Model file for the job. Use its own axes, mm. Face numbers are marked on the shaded views. A direction names the side the tool comes from. Round coordinates to 2 decimals unless told otherwise and drop trailing zeros. Loops run counter-clockwise (first coordinate to the right, second up) from the corner with the lowest first, then second, coordinate; pieces in that order, holes last. Notation, with made-up numbers: (-4.75, 65.5) - (46.25, 65.5) arc R14 cw to (46.25, 81.5) - close; hole circle Ø5 at (85.5, -22.75). An arc over 180 degrees is marked (long way). Answer as a JSON object with one key per item and string values.
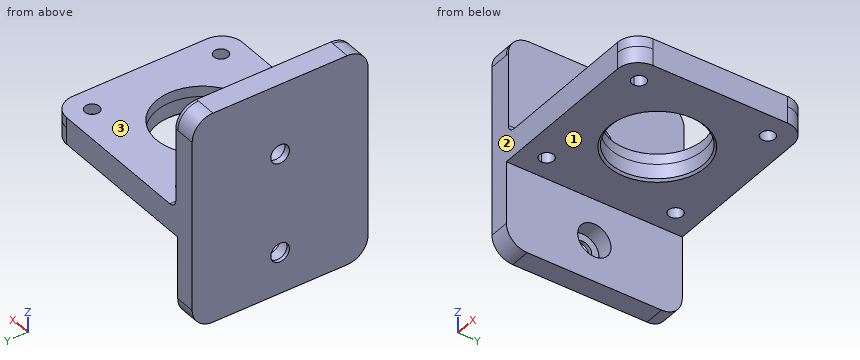
from build123d import *

# Parameters (mm, degrees)
SKETCH1_W                      = 42.3
SKETCH1_H                      = 42.3
BOSS_EXTRUDE1_DEPTH            = 2
M3_CLEARANCE_HOLE1_D           = 3.4
M3_CLEARANCE_HOLE1_CSINK_D     = 3.45
M3_CLEARANCE_HOLE1_CSINK_ANGLE = 90
SKETCH6_R                      = 11.125
CUT_EXTRUDE1_DEPTH             = 5
SKETCH9_W                      = 4.85
SKETCH9_H                      = 42.3
BOSS_EXTRUDE2_DEPTH            = 15
FILLET2_R                      = 5
SKETCH13_W                     = 4.85
SKETCH13_H                     = 42.3
BOSS_EXTRUDE4_DEPTH            = 7
SKETCH14_W                     = 4.85
SKETCH14_H                     = 42.3
BOSS_EXTRUDE5_DEPTH            = 14
CBORE_FOR_M4_SHCS1_D           = 4.5
CBORE_FOR_M4_SHCS1_CBORE_D     = 8
CBORE_FOR_M4_SHCS1_CBORE_DEPTH = 4
FILLET3_R                      = 5
SKETCH19_R                     = 11.125
SKETCH19_R_2                   = 1.725
SKETCH19_R_3                   = 1.7
BOSS_EXTRUDE6_DEPTH            = 2.5
BOSS_EXTRUDE6_DEPTH_BACK       = 4
BOSS_EXTRUDE7_DEPTH            = 0.65
CBORE_FOR_M4_SHCS3_D           = 4.5
CBORE_FOR_M4_SHCS3_CBORE_D     = 8
CBORE_FOR_M4_SHCS3_CBORE_DEPTH = 4
FILLET6_R                      = 2
CHAMFER1_SIZE                  = 0.5


with BuildPart() as part:
    # Sketch1 → Boss-Extrude1 (new body, symmetric)
    with BuildSketch(Plane.XY):
        Rectangle(SKETCH1_W, SKETCH1_H)
    extrude(amount=BOSS_EXTRUDE1_DEPTH, both=True)

    # M3 Clearance Hole1 (through all)
    with Locations(Plane.XY.offset(2)):
        with Locations((-15.5, 15.5), (15.5, 15.5), (15.5, -15.5), (-15.5, -15.5)):
            CounterSinkHole(M3_CLEARANCE_HOLE1_D / 2, M3_CLEARANCE_HOLE1_CSINK_D / 2, counter_sink_angle=M3_CLEARANCE_HOLE1_CSINK_ANGLE)

    # Sketch6 → Cut-Extrude1 (cut, through all)
    with BuildSketch(Plane.XY.offset(2)):
        Circle(SKETCH6_R)
    extrude(amount=-CUT_EXTRUDE1_DEPTH, mode=Mode.SUBTRACT)

    # Sketch9 → Boss-Extrude2 (add, symmetric)
    with BuildSketch(Plane.XY):
        with Locations((-23.575, 0)):
            Rectangle(SKETCH9_W, SKETCH9_H)
    extrude(amount=BOSS_EXTRUDE2_DEPTH, both=True)

    # Fillet2
    fillet2_edges = [part.edges().sort_by_distance(p)[0] for p in [
        (21.15, -21.15, 0),
        (21.15, 21.15, 0),
    ]]
    fillet(fillet2_edges, radius=FILLET2_R)

    # Sketch13 → Boss-Extrude4 (add)
    with BuildSketch(Plane(origin=(0, 0, -15), x_dir=(-1, 0, 0), z_dir=(0, 0, -1))):
        with Locations((23.575, 0)):
            Rectangle(SKETCH13_W, SKETCH13_H)
    extrude(amount=BOSS_EXTRUDE4_DEPTH)

    # Sketch14 → Boss-Extrude5 (add)
    with BuildSketch(Plane.XY.offset(15)):
        with Locations((-23.575, 0)):
            Rectangle(SKETCH14_W, SKETCH14_H)
    extrude(amount=BOSS_EXTRUDE5_DEPTH)

    # CBORE for M4 SHCS1 (through all)
    with Locations(Plane(origin=(-21.15, 0, 0), x_dir=(0, 0, -1), z_dir=(1, 0, 0))):
        with Locations((12, 0)):
            CounterBoreHole(CBORE_FOR_M4_SHCS1_D / 2, CBORE_FOR_M4_SHCS1_CBORE_D / 2, CBORE_FOR_M4_SHCS1_CBORE_DEPTH)

    # Fillet3
    fillet3_edges = [part.edges().sort_by_distance(p)[0] for p in [
        (-23.575, 21.15, -22),
        (-23.575, -21.15, -22),
        (-23.575, -21.15, 29),
        (-23.575, 21.15, 29),
    ]]
    fillet(fillet3_edges, radius=FILLET3_R)

    # Sketch19 → Boss-Extrude6 (add, two sides)
    with BuildSketch(Plane.XY.offset(2)) as boss_extrude6_sk:
        with BuildLine():
            Line((-21.15, -21.15), (16.15, -21.15))
            ThreePointArc((16.15, -21.15), (19.685533906, -19.685533906), (21.15, -16.15))
            Line((21.15, -16.15), (21.15, 16.15))
            ThreePointArc((21.15, 16.15), (19.685533906, 19.685533906), (16.15, 21.15))
            Line((16.15, 21.15), (-21.15, 21.15))
            Line((-21.15, 21.15), (-21.15, -21.15))
        make_face()
        Circle(SKETCH19_R, mode=Mode.SUBTRACT)
        with Locations((15.5, 15.5)):
            Circle(SKETCH19_R_2, mode=Mode.SUBTRACT)
        with Locations((-15.5, 15.5)):
            Circle(SKETCH19_R_2, mode=Mode.SUBTRACT)
        with Locations((-15.5, -15.5)):
            Circle(SKETCH19_R_3, mode=Mode.SUBTRACT)
        with Locations((15.5, -15.5)):
            Circle(SKETCH19_R_3, mode=Mode.SUBTRACT)
    extrude(amount=BOSS_EXTRUDE6_DEPTH)
    extrude(boss_extrude6_sk.sketch, amount=-BOSS_EXTRUDE6_DEPTH_BACK)

    # Sketch21 → Boss-Extrude7 (add)
    with BuildSketch(Plane(origin=(-21.15, 0, 0), x_dir=(0, 0, -1), z_dir=(1, 0, 0))):
        with BuildLine():
            Line((-24, -21.15), (-4.5, -21.15))
            Line((-4.5, -21.15), (-4.5, 21.15))
            Line((-4.5, 21.15), (-24, 21.15))
            ThreePointArc((-24, 21.15), (-27.535533906, 19.685533906), (-29, 16.15))
            Line((-29, 16.15), (-29, -16.15))
            ThreePointArc((-29, -16.15), (-27.535533906, -19.685533906), (-24, -21.15))
        make_face()
    extrude(amount=BOSS_EXTRUDE7_DEPTH)

    # CBORE for M4 SHCS3 (through all)
    with Locations(Plane(origin=(-20.5, 0, 0), x_dir=(0, 0, -1), z_dir=(1, 0, 0))):
        with Locations((-12, 0)):
            CounterBoreHole(CBORE_FOR_M4_SHCS3_D / 2, CBORE_FOR_M4_SHCS3_CBORE_D / 2, CBORE_FOR_M4_SHCS3_CBORE_DEPTH)

    # Fillet6
    fillet6_edges = [part.edges().sort_by_distance(p)[0] for p in [
        (-20.5, 0, 4.5),
    ]]
    fillet(fillet6_edges, radius=FILLET6_R)

    # Chamfer1
    chamfer1_edges = [part.edges().sort_by_distance(p)[0] for p in [
        (-11.125, 0, -2),
    ]]
    chamfer(chamfer1_edges, length=CHAMFER1_SIZE)


solid = part.part
1) Slice it at D-D on y = -13. List the corners of the cut face in (x, z).
Values follow:
{"outline": "(-26, -22) - (-21.15, -22) - (-21.15, -2) - (21.15, -2) - (21.15, 4.5) - (-18.5, 4.5) arc R2 cw to (-20.5, 6.5) - (-20.5, 29) - (-26, 29) - close"}
2) Slice it at C-C on z = -12. List the corners of the cut face in (x, y).
Values follow:
{"outline": "(-26, -21.15) - (-21.15, -21.15) - (-21.15, -4) - (-25.15, -4) - (-25.15, -2.25) - (-26, -2.25) - close; (-26, 2.25) - (-25.15, 2.25) - (-25.15, 4) - (-21.15, 4) - (-21.15, 21.15) - (-26, 21.15) - close"}
3) Tool access for the marked faces 1, 2 and 3: list every direction of +Z, -Z, +X, -X, +Y, -Y with a clear straight run to the whole face (end or side of a thin tool).
Values follow:
{"face 1": "-Z, +X, +Y, -Y", "face 2": "+Z, -Z, +X, -X, -Y", "face 3": "+Z, +X, +Y, -Y"}
4) Slice it at A-A on z = 12. List the corners of the cut face in (x, y).
Values follow:
{"outline": "(-26, -21.15) - (-20.5, -21.15) - (-20.5, -4) - (-24.5, -4) - (-24.5, -2.25) - (-26, -2.25) - close; (-26, 2.25) - (-24.5, 2.25) - (-24.5, 4) - (-20.5, 4) - (-20.5, 21.15) - (-26, 21.15) - close"}
5) Drop flat-ended pins along their axis: P1, Ø10, axis at y = 7.5, z = -14, coming from the +X side; P2, Ø1.5, axis at x = 9, y = 2, coming from the +Z side; P3, Ø6.5, axis at y = -0.5, z = -12, coming from the +X side; P4, Ø5.5, axis at x = -15.5, y = 15.5, coming from the -Z side. Give the stop position or say it passes through.
Values follow:
{"P1": "x = -21.15", "P2": "through", "P3": "x = -25.15", "P4": "z = -2"}
6) Probe probe 1 along X at (y, z) = (15.5, -0.45); probe 2 along Y at (x, z) = (15.5, 3.5) (3 decimals); probe 3 along Y at (x, z) = (-25, 12). List the from-to ranges inside material, lowest first.
Values follow:
{"probe 1": "-26 to -17.2, -13.8 to 13.8, 17.2 to 21.15", "probe 2": "-21.15 to -17.2, -13.8 to 13.775, 17.225 to 21.15", "probe 3": "-21.15 to -2.25, 2.25 to 21.15"}
7) Slice it at B-B on y = 0. Count the separate pieces of the cut face and the enclosed holes in it, then the cut area to 3 significant figures.
Values follow:
{"separate pieces": "4", "enclosed holes": "0", "area": "320 mm²"}
